Design review of the part built by this model. Coordinates are the model's own, in mm. A direction names the side the tool comes from. Coordinates: 2 decimals unless noted, no trailing zeros. Loops run counter-clockwise (first coordinate to the right, second up) from the corner with the lowest first, then second, coordinate; pieces in that order, holes last. Notation, with made-up numbers: M -31,33 L -26,33 A25 ccw -26,46 Z; hole C 46,65 d10. An arc over 180 degrees is marked long. One line per item, written item: value.
```python
from build123d import *

# Parameters (mm, degrees)
F0_R     = 36.3
F1_DEPTH = 10.2
F2_R     = 28
F3_DEPTH = 5
F4_R     = 9.95
F5_DEPTH = 10
F6_R     = 2.5
F7_DEPTH = 15.201
F8_R     = 8.15
F9_DEPTH = 5.201


with BuildPart() as f1:
    # F0 (on Front) → F1 (new body)
    with BuildSketch(Plane.XZ):
        Circle(F0_R)
    extrude(amount=F1_DEPTH)

    # F2 (on face) → F3 (cut)
    with BuildSketch(Plane.XZ.offset(10.2)):
        Circle(F2_R)
    extrude(amount=-F3_DEPTH, mode=Mode.SUBTRACT)

    # F4 (on face) → F5 (join)
    with BuildSketch(Plane.XZ.offset(5.2)):
        Circle(F4_R)
    extrude(amount=F5_DEPTH)

    # F6 (on face) → F7 (cut, through all)
    with BuildSketch(Plane.XZ.offset(15.2)):
        Circle(F6_R)
    extrude(amount=-F7_DEPTH, mode=Mode.SUBTRACT)

    # F8 (on face) → F9 (cut, through all)
    with BuildSketch(Plane.XZ.offset(5.2)):
        with Locations((0, 18.899804)):
            Circle(F8_R)
        with Locations((-17.974782, 5.840361)):
            Circle(F8_R)
        with Locations((-11.109026, -15.290263)):
            Circle(F8_R)
        with Locations((11.109026, -15.290263)):
            Circle(F8_R)
        with Locations((17.974782, 5.840361)):
            Circle(F8_R)
    extrude(amount=-F9_DEPTH, mode=Mode.SUBTRACT)


solid = f1.part
```
(1) Mouldability with a two-part tool opening along Z and no side actions: class faces 3 (the cylindrical face through (5.102, -2.636, -9.782)), 4 (the cylindrical face through (34.624, -5.029, 10.904)), 5 (the flat face through (2, -15.2, -2)) as released by +Z, released by -Z, zero draft, split by the parting line, or undercut.
Reply:
face 3: undercut
face 4: split by the parting line
face 5: zero draft
(2) Tool access review of faces 1 (the cylindrical face through (25.75, -2.64, 8.29)), 2 (the cylindrical face through (-7.9, -10.13, -6.05)): name each direction out of +Z, -Z, +X, -X, +Y, -Y from which nothing blocks a thin tool from reaching the whole face with its end or side.
Reply:
face 1: +Y, -Y
face 2: -Y
(3) We need section D-D on x = 21. State the section outline as (y, z) points, then the cut area to 3 significant figures.
Reply:
outline: M -10.2,-29.61 L 0,-29.61 L 0,-1.73 L -5.2,-1.73 L -5.2,-18.52 L -10.2,-18.52 Z; M -10.2,18.52 L -5.2,18.52 L -5.2,13.41 L 0,13.41 L 0,29.61 L -10.2,29.61 Z
area: 340 mm2
(4) Insertion check: pin 1 (18.5 mm diameter, centred on x = 0, z = 18.9, fed in from +Y); pin 2 (2 mm diameter, centred on x = 0.5, y = -9.5, fed in from +Z); pin 3 (5 mm diameter, centred on x = 3.5, z = -13, fed in from -Y); pin 4 (1 mm diameter, centred on x = -24.5, y = -5.5, fed in from -Z). Each pin has a flat end and moves straight along its axis. Give the tip position at first contact, or say it passes through.
Reply:
pin 1: stops at y = 0
pin 2: stops at z = 36.3
pin 3: stops at y = -5.2
pin 4: stops at z = -27.23
(5) To check wall thickness, follow line 1 along Z through (x, y) = (0, -6); line 2 along X through (y, z) = (-2.25, 1.5); line 3 along Z through (x, y) = (-6, -9). State the ranges of each line that lie inside material, in increasing order. Write a range as [from, to].
Reply:
line 1: z = [-36.3, -28], [-9.95, -2.5], [2.5, 9.95], [28, 36.3]
line 2: x = [-36.27, -24.87], [-11.08, -2], [2, 11.08], [24.87, 36.27]
line 3: z = [-35.8, -27.35], [-7.94, 7.94], [27.35, 35.8]
(6) We need section C-C on y = -7. State the section outline as (x, z) points, then the cut area to 3 significant figures.
Reply:
outline: C 0,0 d72.6; C 0,0 d19.9; hole C 0,0 d56; hole C 0,0 d5
area: 1,970 mm2
(7) We need section B-B on x = 0. State the section outline as (y, z) points, then the cut area to 3 significant figures.
Reply:
outline: M -15.2,-9.95 L -5.2,-9.95 L -5.2,-28 L -10.2,-28 L -10.2,-36.3 L 0,-36.3 L 0,-2.5 L -15.2,-2.5 Z; M -15.2,2.5 L 0,2.5 L 0,10.75 L -5.2,10.75 L -5.2,9.95 L -15.2,9.95 Z; M -10.2,28 L -5.2,28 L -5.2,27.05 L 0,27.05 L 0,36.3 L -10.2,36.3 Z
area: 499 mm2
(8) We need section A-A on z = 0. State the section outline as (x, y) points.
Reply:
outline: M -36.3,-10.2 L -28,-10.2 L -28,-5.2 L -23.66,-5.2 L -23.66,0 L -36.3,0 Z; M -12.29,-5.2 L -9.95,-5.2 L -9.95,-15.2 L -2.5,-15.2 L -2.5,0 L -12.29,0 Z; M 2.5,-15.2 L 9.95,-15.2 L 9.95,-5.2 L 12.29,-5.2 L 12.29,0 L 2.5,0 Z; M 23.66,-5.2 L 28,-5.2 L 28,-10.2 L 36.3,-10.2 L 36.3,0 L 23.66,0 Z
